Model file for the job. Use its own axes, mm. A direction names the side the tool comes from. Give positions to 0.01 mm unless a question says otherwise; leave off trailing zeros. Order: outer loops, then holes, each group sorted by start corner. A loop starts at its lowest first (then second) coordinate and runs counter-clockwise, first axis right, second up. Notation, with made-up numbers: (70, -40) -> (126, -40) arc R30 ccw to (126, -4) -> close; hole circle Ø7 at (43.25, -10.5). An arc over 180 degrees is marked (long way). Answer in a Markdown table with one row per item. Add a question column.
Autodesk Fusion 360 part; units mm, degrees
sketch "mainbase" plane through (0, 0, 0) normal (0, 0, 1) x (1, 0, 0)
  circle A0 centre (0, 0) radius 51
  circle A1 centre (0, 0) radius 46.5
  line L0 (-42.0315, -19.8897) -> (5.9278, -46.1206)
  line L1 (5.9278, -46.1206) -> (45.6951, -8.6144)
  line L2 (45.6951, -8.6144) -> (22.3133, 40.7966)
  line L3 (22.3133, 40.7966) -> (-31.9047, 33.8281)
  line L4 (-31.9047, 33.8281) -> (-42.0315, -19.8897)
  line L5 (-31.9047, 33.8281) -> (0, 0)
  line L6 (0, 0) -> (-42.0315, -19.8897)
  line L7 (5.9278, -46.1206) -> (0, 0)
  line L8 (45.6951, -8.6144) -> (0, 0)
  line L9 (22.3133, 40.7966) -> (0, 0)
  line L10 (-20.0354, 17.8663) -> (-16.8802, 20.3249)
  line L11 (-16.8802, 20.3249) -> (-17.4318, 24.2866)
  line L12 (-17.4318, 24.2866) -> (-21.1386, 25.7899)
  line L13 (-21.1386, 25.7899) -> (-24.2938, 23.3313)
  line L14 (-24.2938, 23.3313) -> (-23.7422, 19.3695)
  line L15 (-23.7422, 19.3695) -> (-20.0354, 17.8663)
  line L16 (19.2822, 26.9195) -> (19.1418, 30.9171)
  line L17 (19.1418, 30.9171) -> (15.6096, 32.7942)
  line L18 (15.6096, 32.7942) -> (12.2178, 30.6738)
  line L19 (12.2178, 30.6738) -> (12.3583, 26.6762)
  line L20 (12.3583, 26.6762) -> (15.8905, 24.7991)
  line L21 (15.8905, 24.7991) -> (19.2822, 26.9195)
  line L22 (30.8937, -9.0267) -> (34.6805, -10.315)
  line L23 (34.6805, -10.315) -> (37.6897, -7.6796)
  line L24 (37.6897, -7.6796) -> (36.912, -3.756)
  line L25 (36.912, -3.756) -> (33.1251, -2.4676)
  line L26 (33.1251, -2.4676) -> (30.116, -5.103)
  line L27 (30.116, -5.103) -> (30.8937, -9.0267)
  line L28 (8.3833, -33.8748) -> (6.093, -30.5954)
  line L29 (6.093, -30.5954) -> (2.1078, -30.9391)
  line L30 (2.1078, -30.9391) -> (0.4128, -34.5622)
  line L31 (0.4128, -34.5622) -> (2.7031, -37.8417)
  line L32 (2.7031, -37.8417) -> (6.6883, -37.498)
  line L33 (6.6883, -37.498) -> (8.3833, -33.8748)
  line L34 (-27.3524, -13.6107) -> (-30.2612, -10.865)
  line L35 (-30.2612, -10.865) -> (-34.0934, -12.0112)
  line L36 (-34.0934, -12.0112) -> (-35.0169, -15.9031)
  line L37 (-35.0169, -15.9031) -> (-32.1082, -18.6488)
  line L38 (-32.1082, -18.6488) -> (-28.2759, -17.5026)
  line L39 (-28.2759, -17.5026) -> (-27.3524, -13.6107)
  line L40 (1.4219, -4.5846) -> (4.6813, -1.0609)
  line L41 (4.6813, -1.0609) -> (3.2594, 3.5237)
  line L42 (3.2594, 3.5237) -> (-1.4219, 4.5846)
  line L43 (-1.4219, 4.5846) -> (-4.6813, 1.0609)
  line L44 (-4.6813, 1.0609) -> (-3.2594, -3.5237)
  line L45 (-3.2594, -3.5237) -> (1.4219, -4.5846)
  point P0 (-20.587, 21.8281)
  point P1 (15.75, 28.7966)
  point P2 (33.9028, -6.3913)
  point P3 (4.3981, -34.2185)
  point P4 (-31.1847, -14.7569)
  dimension "d1" = 102
  dimension "d2" = 93
  dimension "d3" = 46.5
  dimension "d4" = 4
  dimension "d5" = 12
  dimension "d6" = 4
  dimension "d7" = 12
  dimension "d8" = 4
  dimension "d9" = 12
  dimension "d10" = 4
  dimension "d11" = 12
  dimension "d12" = 4
  dimension "d13" = 12
  dimension "d14" = 4.8
extrude "Extrude1" add sketch "mainbase" along normal blind 5 contours A0 | A1 L2 | A1 L3 | L3 L5 L9 L10 L11 L12 L13 L17 L18 L19 L20 L42 L43 | L2 L8 L9 L16 L17 L20 L21 L24 L25 L26 L27 L41 L42 | A1 L1 | L1 L7 L8 L22 L23 L24 L27 L28 L29 L32 L33 L40 L41 L45 | A1 L4 | L4 L5 L6 L10 L13 L14 L15 L34 L35 L36 L37 L43 L44 | L9 L16 L17 L20 L21 | L9 L17 L18 L19 L20 | A1 L0 | L0 L6 L7 L29 L30 L31 L32 L34 L37 L38 L39 L44 L45 | L8 L22 L23 L24 L27 | L8 L24 L25 L26 L27 | L5 L10 L11 L12 L13 | L5 L10 L13 L14 L15 | L7 L29 L30 L31 L32 | L7 L28 L29 L32 L33 | L6 L34 L35 L36 L37 | L6 L34 L37 L38 L39
extrude "Extrude2" cut sketch "mainbase" along normal blind 25 contours L6 L34 L35 L36 L37 | L6 L34 L37 L38 L39
pattern_circular "C-Pattern1" count 4 over 360 about axis through (0, 0, 1.75) along (0, 0, 1) of "Extrude2"
equation "d3 = ( 93 / 2 ) * 1 mm"
Item 1: Two-plate mould, pull along Y, no slides. Class faces 1 (the flat face through (-32.15, -11.43, 2.46)), 2 (the flat face through (-1, -11, 0)), 3 (the cylindrical face through (-11.056, 49.787, 2.465)): pulls with the +Y half, pulls with the -Y half, needs draft (parallel to the pull), parting line crosses it, or undercut.
Item 2: Saw through at D-D on y = -43. List the corners of the cut face in (x, z).
Item 3: Wall check: line 1 (Y direction, x = 31, z = 4.6); line 2 (Y direction, x = 32, z = 2.7); line 3 (X direction, y = 33, z = 1.2). Give the ranges that are in metal, low to high.
Item 4: Which spindle directions (+Z, -Z, +X, -X, +Y, -Y) get a long thin tool onto all of the face, cutting with end or side? Do faces 4 (the flat face through (-12.257, 28.786, 2.465)), 5 (the flat face through (-1, -11, 5)). Say none if no direction does.
Item 5: Saw through at A-A on z = 3.6. Give the number of separate pieces and of enclosed holes in the cut face, plus the area to 3 significant figures.
Item 6: Pin check, flat tips, straight feed: pin 1 Ø3 at (y, z) = (-6.5, 2.5) entering from -X; pin 2 Ø3 at (x, z) = (17.5, 0.5) entering from +Y; pin 3 Ø1 at (y, z) = (-38.5, 1.5) entering from +X. Stop position of each tip, or through.
Item 7: Saw through at B-B on x = 0. List the corners of the cut face in (y, z).
Item 8: Saw through at C-C on x = -39. List the corners of the cut face in (y, z).
Evaluation:
| question | item | result |
|---|---|---|
| 1 | face 1 | undercut |
| 1 | face 2 | needs draft |
| 1 | face 3 | parting line crosses it |
| 2 | outline | (-27.42, 0) -> (27.42, 0) -> (27.42, 5) -> (-27.42, 5) -> close |
| 3 | line 1 | y = -40.5 to 11.09, 18.32 to 40.5 |
| 3 | line 2 | y = -39.71 to 11.39, 18.62 to 39.71 |
| 3 | line 3 | x = -38.88 to -17.81, -11.68 to 38.88 |
| 4 | face 4 | +Z, -Z |
| 4 | face 5 | +Z, +X, -X, +Y, -Y |
| 5 | separate pieces | 1 |
| 5 | enclosed holes | 5 |
| 5 | area | 7,950 mm2 |
| 6 | pin 1 | stops at x = -50.75 |
| 6 | pin 2 | stops at y = 48.43 |
| 6 | pin 3 | stops at x = 34.01 |
| 7 | outline | (-51, 0) -> (-4.26, 0) -> (-4.26, 5) -> (-51, 5) -> close; (4.26, 0) -> (51, 0) -> (51, 5) -> (4.26, 5) -> close |
| 8 | outline | (-32.86, 0) -> (32.86, 0) -> (32.86, 5) -> (-32.86, 5) -> close |
